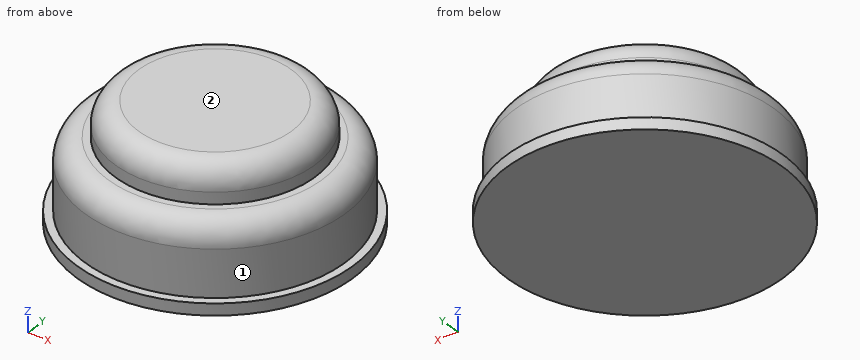
```python
from build123d import *

# Parameters (mm, degrees)
F0_R     = 30.093252
F1_DEPTH = 2.54
F2_R     = 28.342661
F3_DEPTH = 15.24
F4_R     = 5.08
F5_R     = 21.753679
F6_DEPTH = 7.62
F7_R     = 5.08


with BuildPart() as f1:
    # F0 (on Top) → F1 (new body)
    with BuildSketch(Plane.XY):
        Circle(F0_R)
    extrude(amount=F1_DEPTH)

    # F2 (on face) → F3 (join)
    with BuildSketch(Plane.XY.offset(2.54)):
        Circle(F2_R)
    extrude(amount=F3_DEPTH)

    # F4
    f4_edges = [f1.edges().sort_by_distance(p)[0] for p in [
        (-28.342661, 0, 17.78),
    ]]
    fillet(f4_edges, radius=F4_R)

    # F5 (on face) → F6 (join)
    with BuildSketch(Plane.XY.offset(17.78)):
        Circle(F5_R)
    extrude(amount=F6_DEPTH)

    # F7
    f7_edges = [f1.edges().sort_by_distance(p)[0] for p in [
        (-21.753679, 0, 25.4),
    ]]
    fillet(f7_edges, radius=F7_R)


solid = f1.part
```
Input: part model. Units: mm. Frame: model coordinates. Face numbers are marked on the shaded views. Round coordinates to 2 decimals unless told otherwise and drop trailing zeros. Loops run counter-clockwise (first coordinate to the right, second up) from the corner with the lowest first, then second, coordinate; pieces in that order, holes last. Notation, with made-up numbers: (14, 55.25) -> (66, 55.25) arc R21 cw to (66, 94.25) -> close; hole circle Ø1 at (-28.5, -25.75). An arc over 180 degrees is marked (long way). Write each question's results on one line, items separated by ' | '.
1. Section C-C (z = 5.5). Return loops of the section in (x, y), and give its area (3 significant figures).
Geometry results:
outline: circle Ø56.69 at (0, 0) | area: 2,520 mm2
2. Ray query, line 1 (Z direction, x = 12, y = 17); line 2 (Z direction, x = 22.5, y = -4); line 3 (Y direction, x = 23.5, z = 4.75). Return the intervals inside material, ascending. Write a range as from..to.
Geometry results:
line 1: 0..23.27 | line 2: 0..17.78 | line 3: -15.84..15.84
3. Section D-D (z = 13.5). Return loops of the section in (x, y).
Geometry results:
outline: circle Ø56.56 at (0, 0)
4. Section A-A (x = 0). Return loops of the section in (y, z), and give its area (3 significant figures).
Geometry results:
outline: (-30.09, 0) -> (30.09, 0) -> (30.09, 2.54) -> (28.34, 2.54) -> (28.34, 12.7) arc R5.08 ccw to (23.26, 17.78) -> (21.75, 17.78) -> (21.75, 20.32) arc R5.08 ccw to (16.67, 25.4) -> (-16.67, 25.4) arc R5.08 ccw to (-21.75, 20.32) -> (-21.75, 17.78) -> (-23.26, 17.78) arc R5.08 ccw to (-28.34, 12.7) -> (-28.34, 2.54) -> (-30.09, 2.54) -> close | area: 1,330 mm2
5. First-contact query: P1, Ø4, axis at y = -11.5, z = 13, coming from the -X side; P2, Ø2, axis at x = -0.5, z = 4, coming from the +Y side; P3, Ø6, axis at x = 22.5, z = 22.5, coming from the +Y side. Flat tips, straight axial feed; report the tip coordinate or a pass-through.
Geometry results:
P1: x = -26.7 | P2: y = 28.34 | P3: y = 8.97
6. Mould query, pull axis Y, two halves, no side actions, for the marked faces 1 and 2. Classes: +Y half, -Y half, draft (parallel to the pull), parting line (faces both ways), or undercut.
Geometry results:
face 1: parting line | face 2: draft
